from build123d import *

# Parameters (mm, degrees)
F0_W      = 1524
F0_H      = 1016
F1_DEPTH  = 508
F2_W      = 1524
F2_H      = 468.650964
F3_DEPTH  = 254
F4_R      = 254
F1_FACE_W = 1270
F1_FACE_H = 547.349036
F5_DEPTH  = 508
F7_DEPTH  = 1143
F9_DEPTH  = 1143


with BuildPart() as f1:
    # F0 (on Top) → F1 (new body)
    with BuildSketch(Plane.XY):
        with Locations((762, -508)):
            Rectangle(F0_W, F0_H)
    extrude(amount=F1_DEPTH)

    # F2 (on face) → F3 (cut)
    with BuildSketch(Plane.XY.offset(508)):
        with Locations((762, -781.674518)):
            Rectangle(F2_W, F2_H)
    extrude(amount=-F3_DEPTH, mode=Mode.SUBTRACT)

    # F4
    f4_edges = [f1.edges().sort_by_distance(p)[0] for p in [
        (1524, -273.674518, 508),
    ]]
    fillet(f4_edges, radius=F4_R)

    # F1_face (on face) → F5 (join)
    with BuildSketch(Plane(origin=(762, -508, 508), x_dir=(1, 0, 0), z_dir=(0, 0, 1))):
        with Locations((-127, 234.325482)):
            Rectangle(F1_FACE_W, F1_FACE_H)
    extrude(amount=F5_DEPTH)

    # F6 (on face) → F7 (cut)
    with BuildSketch(Plane.XZ.offset(547.349036)):
        with BuildLine():
            Line((0, 1016), (0, 508))
            ThreePointArc((0, 508), (148.789755, 867.210245), (508, 1016))
            Line((508, 1016), (0, 1016))
        make_face()
        with BuildLine():
            ThreePointArc((508, 1016), (867.210245, 867.210245), (1016, 508))
            Line((1016, 508), (1270, 508))
            Line((1270, 508), (1270, 1016))
            Line((1270, 1016), (508, 1016))
        make_face()
    extrude(amount=-F7_DEPTH, mode=Mode.SUBTRACT)

    # F8 (on face) → F9 (cut)
    with BuildSketch(Plane.XZ.offset(547.349036)):
        with BuildLine():
            ThreePointArc((508, 254), (687.605122, 328.394878), (762, 508))
            ThreePointArc((762, 508), (328.394878, 687.605122), (508, 254))
        make_face()
    extrude(amount=-F9_DEPTH, mode=Mode.SUBTRACT)


solid = f1.part
Can you work these out from the model? Positions are in its coordinate system, mm. A direction names the side the tool comes from. Round coordinates to 2 decimals unless told otherwise and drop trailing zeros. Write each loop counter-clockwise with the first axis right and the second up, starting at its lowest first coordinate (ties: lowest second). Pieces come first, ordered by that corner, then holes. Notation, with made-up numbers: M 79.25,10 L 100.25,10 A7 ccw 100.25,20 Z; hole C -34.75,4 d4. An arc over 180 degrees is marked long. Use a Markdown table: item, result.
Item 1: For pin 1 Ø10 at (x, y) = (933.5, -121.5) entering from +Z; pin 2 Ø8 at (y, z) = (-337, 542.5) entering from -X; pin 3 Ø12 at (x, y) = (448.5, -338) entering from -Z; pin 4 Ø4 at (y, z) = (-297, 618.5) entering from +X, each with a flat end and sliding along its axis, tell me the tip position at first contact or that it passes through.
Found:
| item | result |
|---|---|
| pin 1 | stops at z = 793.03 |
| pin 2 | stops at x = 0.92 |
| pin 3 | stops at z = 0 |
| pin 4 | stops at x = 1004.28 |
Item 2: I want a section at D-D (x = 1347). List the corners of the cut face in (y, z) for me.
Found:
| item | result |
|---|---|
| outline | M -1016,0 L 0,0 L 0,496.05 L -547.35,496.05 L -547.35,254 L -1016,254 Z |
Item 3: If I drill on line 1 along Z through (x, y) = (508, -202); line 2 along Z through (x, y) = (107, -609.5); line 3 along Y through (x, z) = (827, 408), over which ranges is the centre line in solid material (lowest first)? Write a range as [from, to].
Found:
| item | result |
|---|---|
| line 1 | z = [0, 254], [762, 1016] |
| line 2 | z = [0, 254] |
| line 3 | y = [-547.35, 0] |
Item 4: Which directions (+Z, -Z, +X, -X, +Y, -Y) give clear straight access to the entire face, cutting with the end or side of a thin tool? Please do faces 1 (the face through (751, -778, 254)), 2 (the face through (1524, -515, 125)), 3 (the face through (1141, -278, 508)).
Found:
| item | result |
|---|---|
| face 1 | +Z, +X, -X, -Y |
| face 2 | +Z, -Z, +X, +Y, -Y |
| face 3 | +Z, +X, +Y, -Y |
Item 5: I want a section at A-A (y = -186.5). List the corners of the cut face in (x, z) for me.
Found:
| item | result |
|---|---|
| outline | M 0,0 L 1524,0 L 1524,254 A254 ccw 1270,508 L 1016,508 A508 ccw 508,1016 A508 ccw 0,508 Z; hole M 508,254 A254 ccw 762,508 A254 ccw long Z |
Item 6: I want a section at C-C (x = 688.5). List the corners of the cut face in (y, z) for me, and give its area (3 significant figures).
Found:
| item | result |
|---|---|
| outline | M -1016,0 L 0,0 L 0,329.29 L -547.35,329.29 L -547.35,254 L -1016,254 Z; M -547.35,686.71 L 0,686.71 L 0,982.85 L -547.35,982.85 Z |
| area | 461,000 mm2 |
Item 7: I want a section at B-B (z = 431). List the corners of the cut face in (x, y) for me, and give its area (3 significant figures).
Found:
| item | result |
|---|---|
| outline | M 0,-547.35 L 265.95,-547.35 L 265.95,0 L 0,0 Z; M 750.05,-547.35 L 1452.17,-547.35 L 1452.17,0 L 750.05,0 Z |
| area | 530,000 mm2 |
